Geometry: final body of the model. Coordinates: model frame, mm. Face numbers are marked on the shaded views. A direction names the side the tool comes from. Give positions to 0.01 mm unless a question says otherwise; leave off trailing zeros. Loops run counter-clockwise (first coordinate to the right, second up) from the corner with the lowest first, then second, coordinate; pieces in that order, holes last. Notation, with made-up numbers: (12.5, 57.5) -> (18.5, 57.5) arc R34 ccw to (18.5, 87.5) -> close; hole circle Ø1 at (5, 59.5). An arc over 180 degrees is marked (long way). One line per question, with ' | ' between items. Start each with the question number.
Item 1: Set-up query: the marked faces 1, 2 and 3. Return all of +Z, -Z, +X, -X, +Y, -Y with unobstructed straight access to the full face (end or side cutting, diameter ignored); none if empty.
Item 2: Section B-B on x = 13. Return loops of the section in (y, z), then the cut area to 3 significant figures.
Item 3: Section C-C on y = 8.25. Return loops of the section in (x, z), then the cut area to 3 significant figures.
Item 4: Material intervals for line 1 along Y through (x, z) = (-16, 11); line 2 along X through (y, z) = (7.25, 10.25); line 3 along X through (y, z) = (6.75, 5.25), sorted ascending. Write a range as [from, to].
Item 5: Pin query (flat end, axial travel): P1, Ø2, axis at x = 4, z = 18, coming from the +Y side; P2, Ø1.5, axis at x = -3.5, z = 5.5, coming from the +Y side; P3, Ø14.5, axis at x = 18, z = 10.5, coming from the -Y side. Return the tip coordinate at first contact, or that it passes through.
Item 6: Section D-D on z = 16.75. Return loops of the section in (x, y) (3 decimals).
Item 7: Section A-A on z = 6.35. Return loops of the section in (x, y) (3 decimals).
from build123d import *

# Parameters (mm, degrees)
BOSS_EXTRUDE2_DEPTH = 25.4
SKETCH2_R           = 2.2225
CUT_EXTRUDE1_DEPTH  = 25.4


with BuildPart() as part:
    # Sketch1 → Boss-Extrude2 (new body)
    with BuildSketch(Plane.XY):
        with BuildLine():
            ThreePointArc((-8.519418994, 9.778156255), (-8.79686691, 11.03471067), (-8.89, 12.318156255))
            Line((-8.89, 12.318156255), (-21.59, 12.318156255))
            Line((-21.59, 12.318156255), (-21.59, 9.778156255))
            Line((-21.59, 9.778156255), (-8.519418994, 9.778156255))
        make_face()
        with BuildLine():
            Line((-6.985, 12.318156255), (-8.89, 12.318156255))
            ThreePointArc((-8.89, 12.318156255), (-8.79686691, 11.03471067), (-8.519418994, 9.778156255))
            ThreePointArc((-8.519418994, 9.778156255), (-5.312791168, 5.190298933), (0, 3.428156255))
            Line((0, 3.428156255), (0, 5.333156255))
            ThreePointArc((0, 5.333156255), (-4.939140867, 7.379015389), (-6.985, 12.318156255))
        make_face()
        with BuildLine():
            ThreePointArc((8.519418994, 9.778156255), (8.79686691, 11.03471067), (8.89, 12.318156255))
            Line((8.89, 12.318156255), (6.985, 12.318156255))
            ThreePointArc((6.985, 12.318156255), (4.939140867, 7.379015389), (0, 5.333156255))
            Line((0, 5.333156255), (0, 3.428156255))
            ThreePointArc((0, 3.428156255), (5.312791168, 5.190298933), (8.519418994, 9.778156255))
        make_face()
        with BuildLine():
            Line((21.59, 12.318156255), (8.89, 12.318156255))
            ThreePointArc((8.89, 12.318156255), (8.79686691, 11.03471067), (8.519418994, 9.778156255))
            Line((8.519418994, 9.778156255), (21.59, 9.778156255))
            Line((21.59, 9.778156255), (21.59, 12.318156255))
        make_face()
    extrude(amount=BOSS_EXTRUDE2_DEPTH)

    # Sketch2 → Cut-Extrude1 (cut)
    with BuildSketch(Plane(origin=(0, 12.318156255, 0), x_dir=(1, 0, 0), z_dir=(0, 1, 0))):
        with Locations(Location((-14.2875, -6.35, 0), (0, 0, 180))):
            Circle(SKETCH2_R)
        with Locations((14.2875, -6.35)):
            Circle(SKETCH2_R)
    extrude(amount=-CUT_EXTRUDE1_DEPTH, mode=Mode.SUBTRACT)


solid = part.part
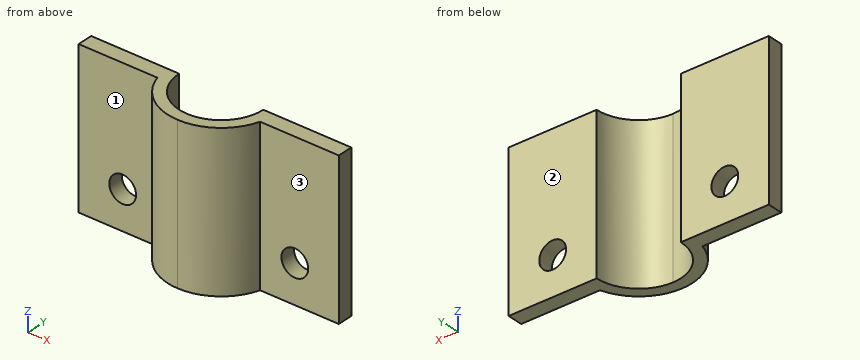
Result sheet:
1) face 1: +Z, -Z, -X, -Y | face 2: +Z, -Z, +X, -X, +Y | face 3: +Z, -Z, +X, -Y
2) outline: (9.78, 0) -> (12.32, 0) -> (12.32, 4.54) -> (9.78, 4.54) -> close; (9.78, 8.16) -> (12.32, 8.16) -> (12.32, 25.4) -> (9.78, 25.4) -> close | area: 55.3 mm²
3) outline: (-7.9, 0) -> (-5.68, 0) -> (-5.68, 25.4) -> (-7.9, 25.4) -> close; (5.68, 0) -> (7.9, 0) -> (7.9, 25.4) -> (5.68, 25.4) -> close | area: 113 mm²
4) line 1: y = [9.78, 12.32] | line 2: x = [-7.3, -4.81], [4.81, 7.3] | line 3: x = [-6.93, -4.22], [4.22, 6.93]
5) P1: stops at y = 7.44 | P2: stops at y = 6.77 | P3: stops at y = 9.78
6) outline: (-21.59, 9.778) -> (-8.519, 9.778) arc R8.89 ccw to (8.519, 9.778) -> (21.59, 9.778) -> (21.59, 12.318) -> (6.985, 12.318) arc R6.985 cw to (-6.985, 12.318) -> (-21.59, 12.318) -> close
7) outline: (-21.59, 9.778) -> (-16.51, 9.778) -> (-16.51, 12.318) -> (-21.59, 12.318) -> close; (-12.065, 9.778) -> (-8.519, 9.778) arc R8.89 ccw to (8.519, 9.778) -> (12.065, 9.778) -> (12.065, 12.318) -> (6.985, 12.318) arc R6.985 cw to (-6.985, 12.318) -> (-12.065, 12.318) -> close; (16.51, 9.778) -> (21.59, 9.778) -> (21.59, 12.318) -> (16.51, 12.318) -> close
